Geometry: final body of the model. Coordinates: model frame, mm. A direction names the side the tool comes from. Round coordinates to 2 decimals unless told otherwise and drop trailing zeros. Loops run counter-clockwise (first coordinate to the right, second up) from the corner with the lowest first, then second, coordinate; pieces in that order, holes last. Notation, with made-up numbers: M -34,-17 L 11,-17 A19 ccw 11,-13 Z; hole C 6.25,26 d4. An arc over 180 degrees is marked long. Answer as a JSON object with one key per item and string values.
from build123d import *

# Parameters (mm, degrees)
F0_R     = 17.5
F1_DEPTH = 5
F2_R     = 12.5
F3_DEPTH = 30
F4_T     = 2.5


# Not quite as in the source:
# - a shell that OpenCascade refuses in one call is made with other operations: the cavity is built on its own and cut out


with BuildPart() as f1:
    # F0 (on Top) → F1 (new body)
    with BuildSketch(Plane.XY):
        Circle(F0_R)
    extrude(amount=F1_DEPTH)

    # F2 (on face) → F3 (join)
    with BuildSketch(Plane.XY.offset(5)):
        Circle(F2_R)
    extrude(amount=F3_DEPTH)

    # F4: shell of thickness 2.5, made by hand


with BuildPart() as f4_core1:
    # F4_t2: copy of F1
    add(f1.part)

    # the walls: a layer under each face that stays
    f4_faces = [f4_core1.faces().sort_by_distance(p)[0] for p in [
        (-17.5, 0, 2.5),
        (0, 0, 0),
        (-11.6666666667, -11.6666666667, 5),
        (-12.5, 0, 20),
    ]]
    thicken(f4_faces, amount=-F4_T, mode=Mode.SUBTRACT)

    # F4_s3 → F4_t4 (revolve, cut)
    with BuildSketch(Plane.XZ):
        Polygon((12.525, 5.025), (12.5, 2.5), (10, 2.5), (10, 5), align=None)
    revolve(axis=Axis((0, 0, 5), (0, 0, 1)), mode=Mode.SUBTRACT)


with BuildPart() as f1_1:
    add(f1.part)

    # what is left inside the walls is the cavity
    f4_cavity = [f4_core1.part.solids().sort_by_distance(p)[0] for p in [
        (-9.975, 0, 13.333333),
    ]]
    add(f4_cavity, mode=Mode.SUBTRACT)


solid = f1_1.part
1) Section query D-D (x = 12). Return the cut outline in (y, z).
Results:
{"outline": "M -12.74,0 L 12.74,0 L 12.74,5 L 3.5,5 L 3.5,35 L -3.5,35 L -3.5,5 L -12.74,5 Z"}
2) Section query B-B (y = 8.5). Return the cut outline in (x, z).
Results:
{"outline": "M -15.3,0 L 15.3,0 L 15.3,5 L 9.17,5 L 9.17,35 L 5.27,35 L 5.27,2.5 L -5.27,2.5 L -5.27,35 L -9.17,35 L -9.17,5 L -15.3,5 Z"}
3) Section query A-A (x = 0). Return the cut outline in (y, z), and give its area (3 significant figures).
Results:
{"outline": "M -17.5,0 L 17.5,0 L 17.5,5 L 12.5,5 L 12.5,35 L 10,35 L 10,2.5 L -10,2.5 L -10,35 L -12.5,35 L -12.5,5 L -17.5,5 Z", "area": "275 mm2"}
4) Reachability of faces 1 (the flat face through (8, -11, 5)), 2 (the flat face through (0, 0, 0)) from +Z, -Z, +X, -X, +Y, -Y: full face, straight path, thin tool, end or side. Return the list, or none.
Results:
{"face 1": "+Z", "face 2": "-Z, +X, -X, +Y, -Y"}
5) Ray query, line 1 (Y direction, x = 0, z = 20); line 2 (Z direction, x = 8.5, y = 13.5); line 3 (Z direction, x = -1, y = 7.5). Return the intervals inside material, ascending.
Results:
{"line 1": "-12.5 to -10, 10 to 12.5", "line 2": "0 to 5", "line 3": "0 to 2.5"}
6) Pull-direction query (X, two-part tool) for faces 3 (the cylindrical face through (-13.887, -10.648, 2.465)), 4 (the flat face through (-0.1, 10.2, 35)), 5 (the cylindrical face through (-2.17, -9.76, 18.98)); classes: +X half, -X half, draft (parallel to the pull), parting line (faces both ways), or undercut.
Results:
{"face 3": "parting line", "face 4": "draft", "face 5": "undercut"}
7) Pin query (flat end, axial travel): P1, Ø3, axis at x = -4.5, y = 12.5, coming from the +Z side; P2, Ø6, axis at x = -5, z = 9.5, coming from the +Y side; P3, Ø10, axis at y = 13, z = 10.5, coming from the +X side; P4, Ø2, axis at x = 2.5, z = 20, coming from the +Y side. Return the tip coordinate at first contact, or that it passes through.
Results:
{"P1": "z = 35", "P2": "y = 12.34", "P3": "x = 9.6", "P4": "y = 12.41"}
8) Section query C-C (z = 7.5). Return the cut outline in (x, y), and give its area (3 significant figures).
Results:
{"outline": "C 0,0 d25; hole C 0,0 d20", "area": "177 mm2"}
